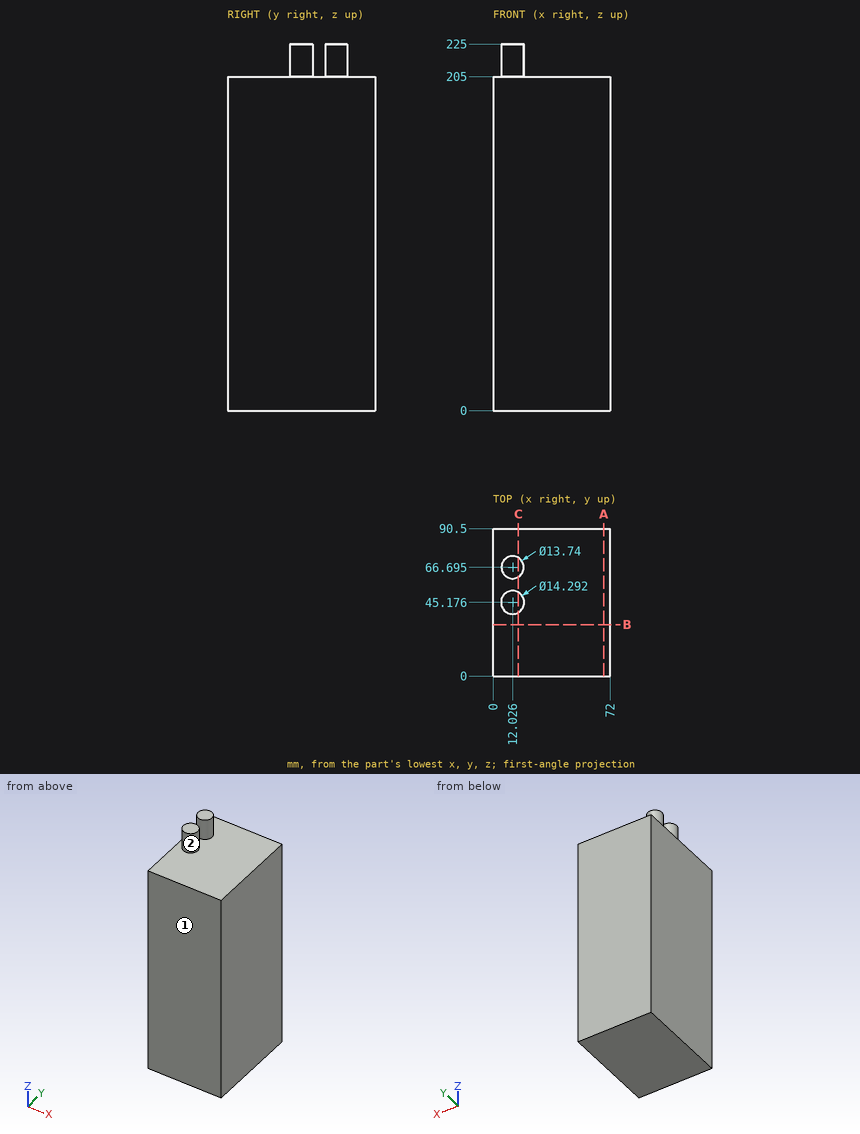
Study the drawing (mm; zero at the part's minimum x, y, z) and answer. A direction names the side the tool comes from. Round coordinates to 2 decimals unless told otherwise and drop trailing zeros. Loops run counter-clockwise (first coordinate to the right, second up) from the corner with the lowest first, then second, coordinate; pieces in that order, holes last. Notation, with made-up numbers: (76.5, -16.75) -> (132.5, -16.75) arc R30 ccw to (132.5, 11.25) -> close; hole circle Ø4 at (-4.75, 56.25). An arc over 180 degrees is marked (long way). Write each question's results on one line, items separated by ' | '. Start each with the question number.
1. Section B-B (y = 31.5) is taken. Determine the outline of the cut face in (x, z), plus the area to 3 significant figures.
2. Given pin 1 Ø2 at (x, y) = (34.5, 34) entering from -Z; pin 2 Ø1.5 at (x, y) = (44.5, 11) entering from +Z, each flat-ended and moving along its own axis, determine where each tip first touches the part or whether it passes through.
3. Find the intervals of material crossed by probe 1 along Z at (x, y) = (49.5, 17), in increasing order. Write a range as from..to.
4. Section C-C (x = 15.5) is taken. Determine the outline of the cut face in (y, z).
5. Section A-A (x = 68) is taken. Determine the outline of the cut face in (y, z), plus the area to 3 significant figures.
6. A tool of negligible diameter and unlimited length cuts with its end or side. For the marked faces 1 and 2, from which of +Z, -Z, +X, -X, +Y, -Y can it reach the whole face along a straight path? Write none if from no direction.
Evaluation:
1) outline: (0, 0) -> (72, 0) -> (72, 205) -> (0, 205) -> close | area: 14,800 mm2
2) pin 1: stops at z = 0 | pin 2: stops at z = 205
3) probe 1: z = 0..205
4) outline: (0, 0) -> (90.5, 0) -> (90.5, 205) -> (72.62, 205) -> (72.62, 225) -> (60.77, 225) -> (60.77, 205) -> (51.42, 205) -> (51.42, 225) -> (38.93, 225) -> (38.93, 205) -> (0, 205) -> close
5) outline: (0, 0) -> (90.5, 0) -> (90.5, 205) -> (0, 205) -> close | area: 18,600 mm2
6) face 1: +Z, -Z, +X, -X, -Y | face 2: +Z
